For this review, take the finished solid that the model builds, in its own axes (mm). Face numbers are marked on the shaded views. A direction names the side the tool comes from. Coordinates: 2 decimals unless noted, no trailing zeros. Loops run counter-clockwise (first coordinate to the right, second up) from the corner with the lowest first, then second, coordinate; pieces in that order, holes last. Notation, with made-up numbers: M 61,33 L 94,33 A32 cw 94,66 Z; hole C -29.75,66.5 d6. An arc over 180 degrees is marked long. Answer as a JSON object with one key per item and string values. Group by question number.
Item 1: Add section B-B (y = 448.5). State the section outline as (x, z) points, then the cut area to 3 significant figures.
Item 2: Add section C-C (y = 105.5). State the section outline as (x, z) points.
Item 3: Insertion check: pin 1 (1 mm diameter, centred on y = 399.5, z = 72.5, fed in from -X); pin 2 (10 mm diameter, centred on y = 349, z = -34, fed in from -X); pin 3 (12 mm diameter, centred on y = 376.5, z = 31.5, fed in from +X). Each pin has a flat end and moves straight along its axis. Give the tip position at first contact, or say it passes through.
Item 4: Wall thickness on L1, parallel to X at y = 577, z = -97; L2, parallel to X at y = 31.5, z = -27; L3, parallel to Z at x = 81, y = 141: over which ranges is each line inside the solid? List them lowest first. Write a range as from..to.
Item 5: Add section A-A (x = 0). State the section outline as (y, z) points, then the cut area to 3 significant figures.
Item 6: Tool access review of the marked faces 1 and 2: name each direction out of +Z, -Z, +X, -X, +Y, -Y from which nothing blocks a thin tool from reaching the whole face with its end or side.
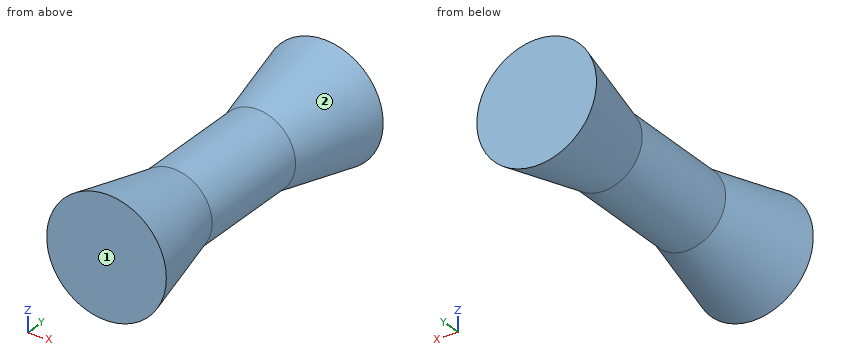
from build123d import *

# Parameters (mm, degrees)
F0_R      = 127
F2_R      = 82.55
F4_R      = 82.55
F5_DEPTH  = 254
F5_FACE_R = 82.55
F7_R      = 127


with BuildPart() as f3:
    # F0 (on Front) → F3 section 0
    with BuildSketch(Plane.XZ):
        Circle(F0_R)
    # F2 (on offset) → F3 section 1
    with BuildSketch(Plane.XZ.offset(-203.2)):
        Circle(F2_R)
    loft()

    # F4 (on offset) → F5 (join)
    with BuildSketch(Plane.XZ.offset(-203.2)):
        Circle(F4_R)
    extrude(amount=-F5_DEPTH)

    # F5_face (on face) → F8 section 0
    with BuildSketch(Plane(origin=(0, 457.2, 0), x_dir=(1, 0, 0), z_dir=(0, 1, 0))):
        Circle(F5_FACE_R)
    # F7 (on offset) → F8 section 1
    with BuildSketch(Plane.XZ.offset(-660.4)):
        Circle(F7_R)
    loft()


solid = f3.part
From the geometry:
{
 "1": {"outline": "C 0,0 d165.1", "area": "21,400 mm²"},
 "2": {"outline": "C 0,0 d207.84"},
 "3": {"pin 1": "stops at x = -40.38", "pin 2": "stops at x = -77.29", "pin 3": "stops at x = 78.51"},
 "4": {"L1": "x = -49.18..49.18", "L2": "x = -117.04..117.04", "L3": "z = -51.82..51.82"},
 "5": {"outline": "M 0,-127 L 203.2,-82.55 L 457.2,-82.55 L 660.4,-127 L 660.4,127 L 457.2,82.55 L 203.2,82.55 L 0,127 Z", "area": "127,000 mm²"},
 "6": {"face 1": "+Z, -Z, +X, -X, -Y", "face 2": "none"}
}
